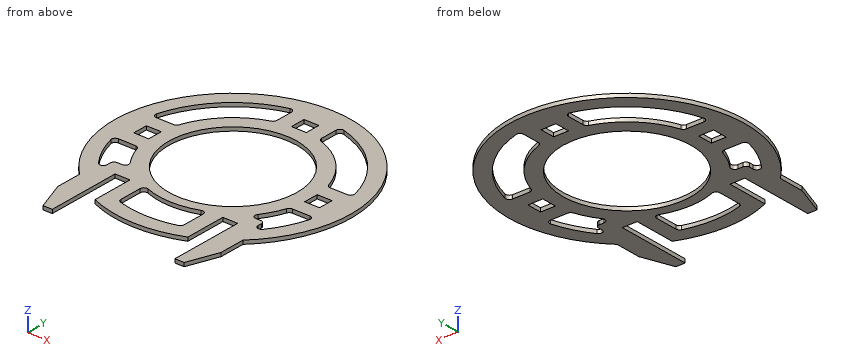
```python
from build123d import *

# Parameters (mm, degrees)
ESQUISSE1_R        = 172
ESQUISSE1_W        = 40
ESQUISSE1_H        = 40
BOSS_EXTRU_1_DEPTH = 10
CONG_1_R           = 10


with BuildPart() as part:
    # Esquisse1 → Boss.-Extru.1 (new body)
    with BuildSketch(Plane.XY):
        with BuildLine():
            Line((220, -228.230147001), (220, -297.575677416))
            Line((220, -297.575677416), (190, -380))
            Line((190, -380), (165, -380))
            Line((165, -380), (165, -180))
            Line((165, -180), (125, -180))
            Line((125, -180), (125, -291.314263297))
            ThreePointArc((125, -291.314263297), (0, -317), (-125, -291.314263297))
            Line((-125, -291.314263297), (-125, -180))
            Line((-125, -180), (-165, -180))
            Line((-165, -180), (-165, -380))
            Line((-165, -380), (-190, -380))
            Line((-190, -380), (-220, -297.575677416))
            Line((-220, -297.575677416), (-220, -228.230147001))
            ThreePointArc((-220, -228.230147001), (0, 317), (220, -228.230147001))
        make_face()
        Circle(ESQUISSE1_R, mode=Mode.SUBTRACT)
        with Locations((230, 0)):
            Rectangle(ESQUISSE1_W, ESQUISSE1_H, mode=Mode.SUBTRACT)
        with BuildLine():
            Line((270.423741561, 60), (203.332240434, 60))
            ThreePointArc((203.332240434, 60), (149.906637612, 149.906637612), (60, 203.332240434))
            Line((60, 203.332240434), (60, 270.423741561))
            ThreePointArc((60, 270.423741561), (195.868578389, 195.868578389), (270.423741561, 60))
        make_face(mode=Mode.SUBTRACT)
        with BuildLine():
            Line((-60, 270.423741561), (-60, 203.332240434))
            ThreePointArc((-60, 203.332240434), (-149.906637612, 149.906637612), (-203.332240434, 60))
            Line((-203.332240434, 60), (-270.423741561, 60))
            ThreePointArc((-270.423741561, 60), (-195.868578389, 195.868578389), (-60, 270.423741561))
        make_face(mode=Mode.SUBTRACT)
        with BuildLine():
            Line((203.332240434, -60), (270.423741561, -60))
            ThreePointArc((270.423741561, -60), (245.385741824, -128.510068513), (203.332240434, -188.109010948))
            Line((203.332240434, -188.109010948), (203.332240434, -140))
            Line((203.332240434, -140), (159.197989937, -140))
            ThreePointArc((159.197989937, -140), (185.626081097, -102.405849524), (203.332240434, -60))
        make_face(mode=Mode.SUBTRACT)
        with Locations((-230, 0)):
            Rectangle(ESQUISSE1_W, ESQUISSE1_H, mode=Mode.SUBTRACT)
        with Locations((0, 230)):
            Rectangle(ESQUISSE1_W, ESQUISSE1_H, mode=Mode.SUBTRACT)
        with BuildLine():
            Line((-85, -180), (-85, -263.636112853))
            ThreePointArc((-85, -263.636112853), (0, -277), (85, -263.636112853))
            Line((85, -263.636112853), (85, -180))
            ThreePointArc((85, -180), (0, -199.060292374), (-85, -180))
        make_face(mode=Mode.SUBTRACT)
        with BuildLine():
            Line((-203.332240434, -60), (-270.423741561, -60))
            ThreePointArc((-270.423741561, -60), (-245.385741824, -128.510068513), (-203.332240434, -188.109010948))
            Line((-203.332240434, -188.109010948), (-203.332240434, -140))
            Line((-203.332240434, -140), (-159.197989937, -140))
            ThreePointArc((-159.197989937, -140), (-185.626081097, -102.405849524), (-203.332240434, -60))
        make_face(mode=Mode.SUBTRACT)
    extrude(amount=BOSS_EXTRU_1_DEPTH)

    # Congé1
    cong_1_edges = [part.edges().sort_by_distance(p)[0] for p in [
        (270.423741561, 60, 5),
        (60, 270.423741561, 5),
        (60, 203.332240434, 5),
        (203.332240434, 60, 5),
        (-60, 270.423741561, 5),
        (-270.423741561, 60, 5),
        (-203.332240434, 60, 5),
        (-60, 203.332240434, 5),
        (85, -180, 5),
        (-85, -180, 5),
        (-85, -263.636112853, 5),
        (85, -263.636112853, 5),
        (203.332240434, -60, 5),
        (159.197989937, -140, 5),
        (203.332240434, -140, 5),
        (203.332240434, -188.109010948, 5),
        (270.423741561, -60, 5),
        (-159.197989937, -140, 5),
        (-203.332240434, -60, 5),
        (-270.423741561, -60, 5),
        (-203.332240434, -188.109010948, 5),
        (-203.332240434, -140, 5),
    ]]
    fillet(cong_1_edges, radius=CONG_1_R)


solid = part.part
```
Source: CAD feature listing. Evaluate the final solid. Frame: model axes, mm. Coordinates: 2 decimals unless noted, no trailing zeros. Loops run counter-clockwise (first coordinate to the right, second up) from the corner with the lowest first, then second, coordinate; pieces in that order, holes last. Notation, with made-up numbers: M -36,10 L 14,10 A20 cw 14,49 Z; hole C -1.5,77.25 d4. An arc over 180 degrees is marked long. Use a Markdown table: item, result. Add a question column.
Q1. Section query B-B, the plane x = 0. Return loops of the section in (y, z), and give its area (3 significant figures).
Q2. Section query A-A, the plane y = -237. Return loops of the section in (x, z).
Q3. Section query C-C, the plane x = -101. Return loops of the section in (y, z), and give its area (3 significant figures).
Q4. First-contact query: pin 1 (1 mm diameter, centred on y = -286.5, z = 4, fed in from +X); pin 2 (1 mm diameter, centred on y = -207.5, z = 1.5, fed in from -X); pin 3 (12 mm diameter, centred on x = -33.5, y = -193.5, fed in from -Z); pin 4 (3 mm diameter, centred on y = 223.5, z = 5.5, fed in from +X). Flat tips, straight axial feed; report the tip coordinate or a pass-through.
Q5. Material intervals for L1, parallel to Y at x = 0, z = 2.25; L2, parallel to X at y = -246.5, z = 4.5; L3, parallel to X at y = 186.5, z = 7, sorted ascending.
Q6. Section query D-D, the plane z = 6.25. State how many separate pieces and enclosed holes the cut face has, and give its area (3 significant figures).
Result:
| question | item | result |
|---|---|---|
| 1 | outline | M -317,0 L -277,0 L -277,10 L -317,10 Z; M -199.06,0 L -172,0 L -172,10 L -199.06,10 Z; M 172,0 L 210,0 L 210,10 L 172,10 Z; M 250,0 L 317,0 L 317,10 L 250,10 Z |
| 1 | area | 1,720 mm2 |
| 2 | outline | M -220,0 L -165,0 L -165,10 L -220,10 Z; M -125,0 L -85,0 L -85,10 L -125,10 Z; M 85,0 L 125,0 L 125,10 L 85,10 Z; M 165,0 L 220,0 L 220,10 L 165,10 Z |
| 3 | outline | M -300.48,0 L -139.22,0 L -139.22,10 L -300.48,10 Z; M 139.22,0 L 186.39,0 L 186.39,10 L 139.22,10 Z; M 257.93,0 L 300.48,0 L 300.48,10 L 257.93,10 Z |
| 3 | area | 2,510 mm2 |
| 4 | pin 1 | stops at x = 220 |
| 4 | pin 2 | stops at x = -240.08 |
| 4 | pin 3 | stops at z = 0 |
| 4 | pin 4 | stops at x = 226.29 |
| 5 | L1 | y = -317 to -277, -199.06 to -172, 172 to 210, 250 to 317 |
| 5 | L2 | x = -220 to -165, -125 to -85, 85 to 125, 165 to 220 |
| 5 | L3 | x = -256.33 to -204.81, -100.81 to 100.81, 204.81 to 256.33 |
| 6 | separate pieces | 1 |
| 6 | enclosed holes | 9 |
| 6 | area | 161,000 mm2 |
